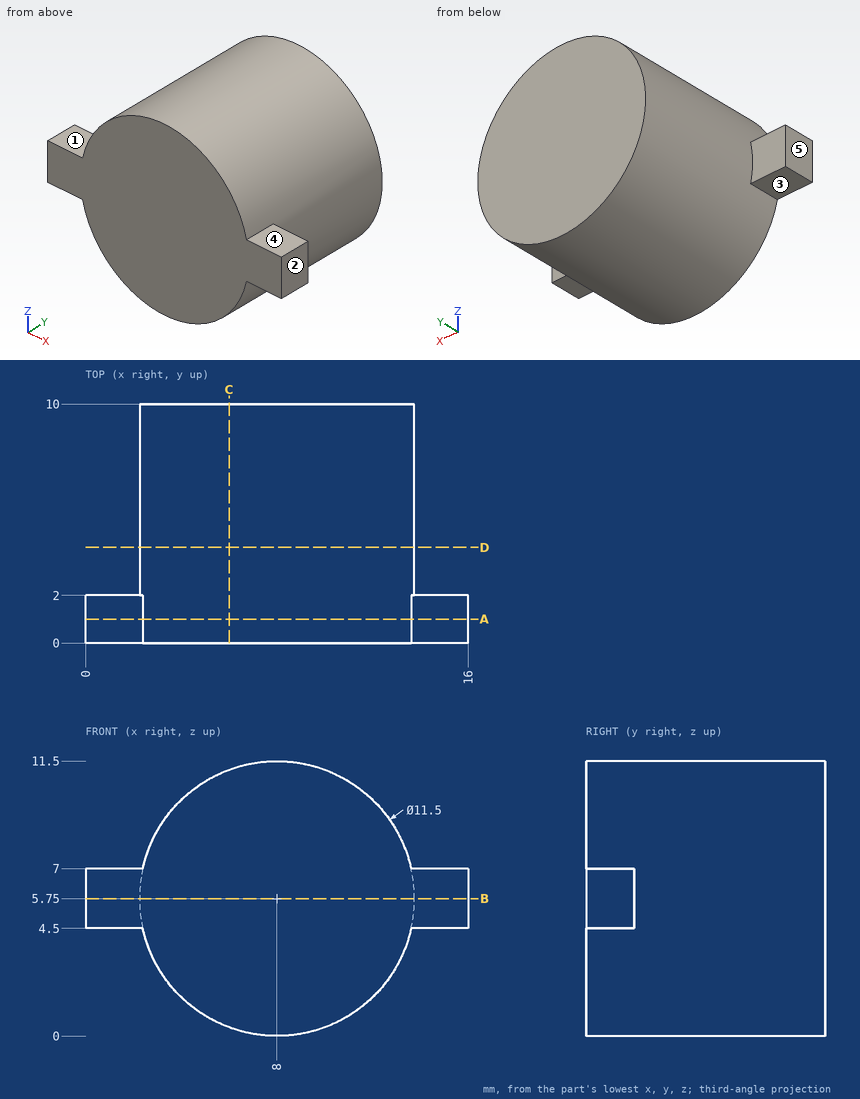
Print and shaded views of the part. All mm, measured from the part's lowest x, y and z. A direction names the side the tool comes from. Round coordinates to 2 decimals unless told otherwise and drop trailing zeros. Order: outer loops, then holes, each group sorted by start corner. A loop starts at its lowest first (then second) coordinate and runs counter-clockwise, first axis right, second up. Notation, with made-up numbers: (-17, -11) - (-5, -11) arc R15 ccw to (-5, 17) - close; hole circle Ø7 at (45.25, -28). An arc over 180 degrees is marked (long way). Use a Markdown table: item, result.
1) Saw through at B-B on z = 5.75. Write the cut outline in (x, y).
Recorded:
| item | result |
|---|---|
| outline | (0, 0) - (16, 0) - (16, 2) - (13.75, 2) - (13.75, 10) - (2.25, 10) - (2.25, 2) - (0, 2) - close |
2) Flat gauge pins, fed straight in: pin 1 Ø0.7 at (x, z) = (1.5, 5) entering from +Y; pin 2 Ø1 at (x, y) = (14.5, 0.5) entering from -Z; pin 3 Ø5 at (x, y) = (14, 4) entering from +Z. Where does each tip first touch, or does it go through?
Recorded:
| item | result |
|---|---|
| pin 1 | stops at y = 2 |
| pin 2 | stops at z = 4.5 |
| pin 3 | stops at z = 10.31 |
3) Tool access for the marked faces 4 and 5: list every direction of +Z, -Z, +X, -X, +Y, -Y with a clear straight run to the whole face (end or side of a thin tool).
Recorded:
| item | result |
|---|---|
| face 4 | +Z, +X, +Y, -Y |
| face 5 | +Z, -Z, -X, +Y, -Y |
4) Saw through at C-C on x = 6. Write the cut outline in (y, z).
Recorded:
| item | result |
|---|---|
| outline | (0, 0.36) - (10, 0.36) - (10, 11.14) - (0, 11.14) - close |
5) Saw through at A-A on y = 1. Write the cut outline in (x, z), and give its area (3 significant figures).
Recorded:
| item | result |
|---|---|
| outline | (0, 4.5) - (2.39, 4.5) arc R5.75 ccw to (13.61, 4.5) - (16, 4.5) - (16, 7) - (13.61, 7) arc R5.75 ccw to (2.39, 7) - (0, 7) - close |
| area | 115 mm² |
6) Wall check: L1, parallel to X at y = 1.5, z = 10.5; L2, parallel to X at y = 1, z = 3; L3, parallel to Z at x = 12, y = 7.75. Give the ranges that are in metal, low to high.
Recorded:
| item | result |
|---|---|
| L1 | x = 4.76 to 11.24 |
| L2 | x = 2.95 to 13.05 |
| L3 | z = 1.62 to 9.88 |
7) Saw through at D-D on y = 4. Write the cut outline in (x, z), and give its area (3 significant figures).
Recorded:
| item | result |
|---|---|
| outline | circle Ø11.5 at (8, 5.75) |
| area | 104 mm² |
8) Pull direction Z, two halves, no side cores. Call the marked faces 1, 2 and 3: pulls with the +Z half, pulls with the -Z half, needs draft (parallel to the pull), parting line crosses it, or undercut.
Recorded:
| item | result |
|---|---|
| face 1 | pulls with the +Z half |
| face 2 | needs draft |
| face 3 | pulls with the -Z half |
